Geometry: see drawing. Coordinates: mm, zero at the bounding-box minimum. A direction names the side the tool comes from. Coordinates: 2 decimals unless noted, no trailing zeros. Order: outer loops, then holes, each group sorted by start corner. A loop starts at its lowest first (then second) coordinate and runs counter-clockwise, first axis right, second up.
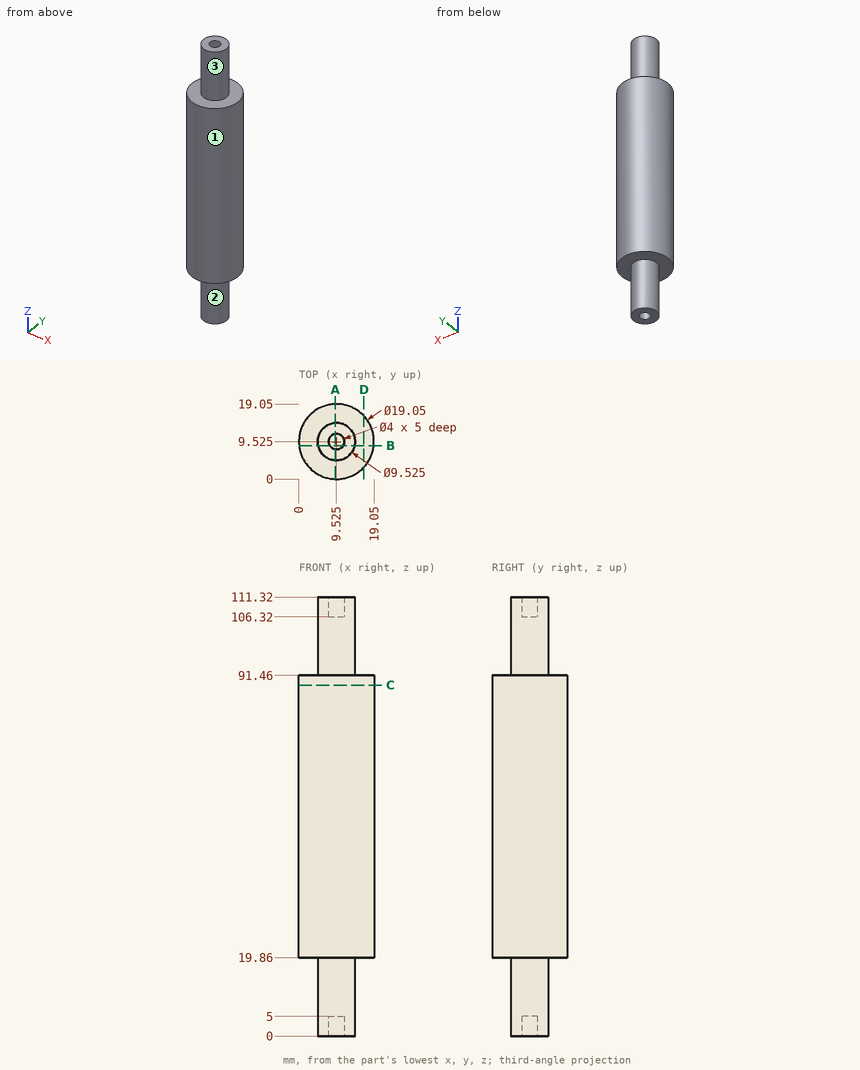
Q1. Set-up query: the marked faces 1, 2 and 3. Return all of +Z, -Z, +X, -X, +Y, -Y with unobstructed straight access to the full face (end or side cutting, diameter ignored); none if empty.
Solutions:
face 1: +Z, -Z
face 2: -Z
face 3: +Z
Q2. Section query D-D on x = 16.5. Output: boundary loops of the cut face in (y, z).
Solutions:
outline: (3.04, 19.86) - (16.01, 19.86) - (16.01, 91.46) - (3.04, 91.46) - close
Q3. Section query C-C on z = 89. Output: boundary loops of the cut face in (x, y) (3 decimals).
Solutions:
outline: circle Ø19.05 at (9.525, 9.525)
Q4. Material intervals for line 1 along Z through (x, y) = (8.25, 15.5); line 2 along Z through (x, y) = (8.5, 8); line 3 along X through (y, z) = (9.75, 13.5), sorted ascending.
Solutions:
line 1: z = 19.86 to 91.46
line 2: z = 5 to 106.32
line 3: x = 4.77 to 14.28
Q5. Section query B-B on y = 8.5. Output: boundary loops of the cut face in (x, z).
Solutions:
outline: (0.06, 19.86) - (4.87, 19.86) - (4.87, 0) - (7.81, 0) - (7.81, 5) - (11.24, 5) - (11.24, 0) - (14.18, 0) - (14.18, 19.86) - (18.99, 19.86) - (18.99, 91.46) - (14.18, 91.46) - (14.18, 111.32) - (11.24, 111.32) - (11.24, 106.32) - (7.81, 106.32) - (7.81, 111.32) - (4.87, 111.32) - (4.87, 91.46) - (0.06, 91.46) - close
Q6. Section query A-A on x = 9.25. Output: boundary loops of the cut face in (y, z).
Solutions:
outline: (0, 19.86) - (4.77, 19.86) - (4.77, 0) - (7.54, 0) - (7.54, 5) - (11.51, 5) - (11.51, 0) - (14.28, 0) - (14.28, 19.86) - (19.05, 19.86) - (19.05, 91.46) - (14.28, 91.46) - (14.28, 111.32) - (11.51, 111.32) - (11.51, 106.32) - (7.54, 106.32) - (7.54, 111.32) - (4.77, 111.32) - (4.77, 91.46) - (0, 91.46) - close
Q7. Pin query (flat end, axial travel): P1, Ø1.5, axis at x = 12.5, y = 8, coming from the -Z side; P2, Ø4, axis at x = 7, z = 39, coming from the +Y side; P3, Ø3, axis at x = 9.525, y = 9.525, coming from the +Z side; P4, Ø6, axis at y = 14.5, z = 86, coming from the -X side. Return the tip coordinate at first contact, or that it passes through.
Solutions:
P1: stops at z = 0
P2: stops at y = 19.04
P3: stops at z = 106.32
P4: stops at x = 0.21
